Verification items for the finished model (mm, model axes). Coordinates: 2 decimals unless noted, no trailing zeros. Order: outer loops, then holes, each group sorted by start corner. A loop starts at its lowest first (then second) coordinate and runs counter-clockwise, first axis right, second up. Notation, with made-up numbers: M 53,28 L 73,28 A29 cw 73,54 Z; hole C 74.5,13.5 d2. An arc over 180 degrees is marked long. Return JSON: item names as keys, results as strings. Group by question number.
Q1. Thickness scan on probe 1 along Z at (x, y) = (-68, -8.25); probe 2 along X at (y, z) = (-7.25, 9); probe 3 along X at (y, z) = (-5.5, -53). Record the ranges inside material, lowest first.
Q2. Mould release check, pull along X, two halves, no side actions. Record for faces 1 (the face through (-106.14, -2.01, -52.54)), 2 (the face through (-97.832, -6.332, 43.282)), 3 (the face through (-66.504, -4.833, -28.468)): pulls with the +X half, pulls with the -X half, needs draft (parallel to the pull), parting line crosses it, or undercut.
Q3. Go/stop test with flat-tipped pins: pin 1 Ø1 at (x, y) = (-92.5, -5.5) entering from +Z; pin 2 Ø1.5 at (y, z) = (-1.5, -23) entering from +X. Record where each tip stops, or that it passes through.
Q4. Section check B-B, the plane y = -9.75. Enter the section's corners in (x, z).
Q5. Section check A-A, the plane y = -2.25. Enter the section's corners in (x, z), then the cut area to 3 significant figures.
from build123d import *

# Parameters (mm, degrees)
F0_R         = 57.9360533335
F2_DEPTH     = 12.7
F3_D         = 48.26
F5_D         = 33.02
F6_T2_ANGLE  = 283.4727948919
F6_T4_ANGLE  = 86.0712547595
F6_T6_ANGLE  = 107.4118170834
F6_T8_ANGLE  = 267.462303274
F6_T10_ANGLE = 277.2145700269
F6_T12_ANGLE = 103.4165555336
F6_T16_ANGLE = 107.4118170834
F6_T18_ANGLE = 283.4727948919
F6_T20_ANGLE = 277.2145700269
F6_T22_ANGLE = 86.0712547595
F6_T24_ANGLE = 103.4165555336
F6_T26_ANGLE = 267.462303274


# Not quite as in the source:
# - a fillet or chamfer that OpenCascade refuses, or shapes differently, is made with other operations: its cross-section is extruded or revolved along the edge and cut away or added


with BuildPart() as f2:
    # F0 (on Front) → F2 (new body)
    with BuildSketch(Plane.XZ):
        with Locations((-72.7998018265, -8.9674890041)):
            Circle(F0_R)
    extrude(amount=F2_DEPTH)

    # F3 (through all)
    with Locations(Plane(origin=(0, 0, 0), x_dir=(1, 0, 0), z_dir=(0, 1, 0))):
        with Locations((-45.7866154611, -28.1515028328), (-120.4445809126, 8.0565353855), (-60.4006908834, 52.0677864552)):
            Hole(F3_D / 2)

    # F5 (through all)
    with Locations(Plane(origin=(0, 0, 0), x_dir=(1, 0, 0), z_dir=(0, 1, 0))):
        with Locations((-74.9381706119, 4.8889117315)):
            Hole(F5_D / 2)

    # F6: chamfer of 5.08 on 14 edges, made by hand

    # F6_s1 → F6_t2 (revolve, cut)
    with BuildSketch(Plane(origin=(-33.5431340109, 0, 13.6983383479), x_dir=(0, 1, 0), z_dir=(0.9257774909, 0, -0.3780688263))):
        Polygon((-7.62, -95.1688030077), (-12.7, -100.2488030077), (-12.7, -95.1688030077), align=None)
    revolve(axis=Axis((-60.4006908834, -12.7, -52.0677864552), (0, 1, 0)), revolution_arc=F6_T2_ANGLE, mode=Mode.SUBTRACT)

    # F6_s3 → F6_t4 (revolve, cut)
    with BuildSketch(Plane(origin=(-0.6504253771, 0, 3.7035474889), x_dir=(0, 1, 0), z_dir=(-0.1729749681, 0, 0.9849262208))):
        Polygon((-12.7, 126.1096381457), (-7.62, 131.1896381457), (-12.7, 131.1896381457), align=None)
    revolve(axis=Axis((-72.7998018265, -12.7, -8.9674890041), (0, -1, 0)), revolution_arc=F6_T4_ANGLE, mode=Mode.SUBTRACT)

    # F6_s5 → F6_t6 (revolve, cut)
    with BuildSketch(Plane(origin=(-29.9879926822, 0, 31.6264228209), x_dir=(0, 1, 0), z_dir=(-0.6880604052, 0, 0.7256534151))):
        Polygon((-7.62, 1.0615455961), (-12.7, 6.1415455961), (-12.7, 1.0615455961), align=None)
    revolve(axis=Axis((-72.7998018265, -12.7, -8.9674890041), (0, 1, 0)), revolution_arc=F6_T6_ANGLE, mode=Mode.SUBTRACT)

    # F6_s7 → F6_t8 (revolve, cut)
    with BuildSketch(Plane(origin=(-69.201107614, 0, -63.7135426846), x_dir=(0, 1, 0), z_dir=(-0.7356739262, 0, -0.6773358652))):
        Polygon((-12.7, -104.8644514037), (-7.62, -99.7844514037), (-12.7, -99.7844514037), align=None)
    revolve(axis=Axis((-120.4445809126, -12.7, -8.0565353855), (0, 1, 0)), revolution_arc=F6_T8_ANGLE, mode=Mode.SUBTRACT)

    # F6_s9 → F6_t10 (revolve, cut)
    with BuildSketch(Plane(origin=(-8.1423267798, 0, 36.5399201696), x_dir=(0, 1, 0), z_dir=(-0.2174992035, 0, 0.9760604984))):
        Polygon((-12.7, 9.3575772605), (-7.62, 14.4375772605), (-12.7, 14.4375772605), align=None)
    revolve(axis=Axis((-45.7866154611, -12.7, 28.1515028328), (0, 1, 0)), revolution_arc=F6_T10_ANGLE, mode=Mode.SUBTRACT)

    # F6_s11 → F6_t12 (revolve, cut)
    with BuildSketch(Plane(origin=(-55.7502574842, 0, 26.6710376642), x_dir=(0, 1, 0), z_dir=(0.9020846433, 0, -0.4315591458))):
        Polygon((-12.7, 13.3491989235), (-7.62, 18.4291989235), (-12.7, 18.4291989235), align=None)
    revolve(axis=Axis((-72.7998018265, -12.7, -8.9674890041), (0, -1, 0)), revolution_arc=F6_T12_ANGLE, mode=Mode.SUBTRACT)

    # F6_s13 → F6_t14 (revolve, cut)
    with BuildSketch(Plane.XY.offset(-4.8889117315)):
        Polygon((-53.3481706119, -12.7), (-58.4281706119, -7.62), (-58.4281706119, -12.7), align=None)
    revolve(axis=Axis((-74.9381706119, -12.7, -4.8889117315), (0, 1, 0)), mode=Mode.SUBTRACT)

    # F6_s15 → F6_t16 (revolve, cut)
    with BuildSketch(Plane(origin=(-62.2843162467, 0, -30.4655418629), x_dir=(0, 1, 0), z_dir=(-0.8982965238, 0, -0.4393897533))):
        Polygon((-5.08, 34.004030567), (0, 28.924030567), (0, 34.004030567), align=None)
    revolve(axis=Axis((-72.7998018265, 0, -8.9674890041), (0, -1, 0)), revolution_arc=F6_T16_ANGLE, mode=Mode.SUBTRACT)

    # F6_s17 → F6_t18 (revolve, cut)
    with BuildSketch(Plane(origin=(-45.2248879791, 0, -62.9674495541), x_dir=(0, 1, 0), z_dir=(-0.5833556277, 0, -0.8122168501))):
        Polygon((0, 10.5255773581), (-5.08, 5.4455773581), (0, 5.4455773581), align=None)
    revolve(axis=Axis((-60.4006908834, 0, -52.0677864552), (0, -1, 0)), revolution_arc=F6_T18_ANGLE, mode=Mode.SUBTRACT)

    # F6_s19 → F6_t20 (revolve, cut)
    with BuildSketch(Plane(origin=(-8.1423267798, 0, 36.5399201696), x_dir=(0, 1, 0), z_dir=(-0.2174992035, 0, 0.9760604984))):
        Polygon((0, 9.3575772605), (-5.08, 14.4375772605), (0, 14.4375772605), align=None)
    revolve(axis=Axis((-45.7866154611, 0, 28.1515028328), (0, 1, 0)), revolution_arc=F6_T20_ANGLE, mode=Mode.SUBTRACT)

    # F6_s21 → F6_t22 (revolve, cut)
    with BuildSketch(Plane(origin=(-0.6504253771, 0, 3.7035474889), x_dir=(0, 1, 0), z_dir=(-0.1729749681, 0, 0.9849262208))):
        Polygon((0, 126.1096381457), (-5.08, 131.1896381457), (0, 131.1896381457), align=None)
    revolve(axis=Axis((-72.7998018265, 0, -8.9674890041), (0, -1, 0)), revolution_arc=F6_T22_ANGLE, mode=Mode.SUBTRACT)

    # F6_s23 → F6_t24 (revolve, cut)
    with BuildSketch(Plane(origin=(-55.7502574842, 0, 26.6710376642), x_dir=(0, 1, 0), z_dir=(0.9020846433, 0, -0.4315591458))):
        Polygon((0, 13.3491989235), (-5.08, 18.4291989235), (0, 18.4291989235), align=None)
    revolve(axis=Axis((-72.7998018265, 0, -8.9674890041), (0, -1, 0)), revolution_arc=F6_T24_ANGLE, mode=Mode.SUBTRACT)

    # F6_s25 → F6_t26 (revolve, cut)
    with BuildSketch(Plane(origin=(-56.5588266789, 0, 56.2173150628), x_dir=(0, 1, 0), z_dir=(-0.7092448082, 0, 0.7049622699))):
        Polygon((0, 119.832941055), (-5.08, 114.752941055), (0, 114.752941055), align=None)
    revolve(axis=Axis((-120.4445809126, 0, -8.0565353855), (0, -1, 0)), revolution_arc=F6_T26_ANGLE, mode=Mode.SUBTRACT)

    # F6_s27 → F6_t28 (revolve, cut)
    with BuildSketch(Plane.XY.offset(-4.8889117315)):
        Polygon((-53.3481706119, 0), (-58.4281706119, -5.08), (-58.4281706119, 0), align=None)
    revolve(axis=Axis((-74.9381706119, 0, -4.8889117315), (0, 1, 0)), mode=Mode.SUBTRACT)


solid = f2.part
Numbers:
{
 "1": {"probe 1": "z = -28.5 to -20.56, 10.78 to 17.21, 39.09 to 48.14", "probe 2": "x = -103.38 to -83.86, -66.01 to -60.47, -31.11 to -17.72", "probe 3": "x = -110.45 to -84.51, -36.29 to -35.15"},
 "2": {"face 1": "pulls with the -X half", "face 2": "parting line crosses it", "face 3": "undercut"},
 "3": {"pin 1": "stops at z = 45.69", "pin 2": "stops at x = -19.49"},
 "4": {"outline": "M -122.56,-34.23 A55.81 ccw -83.97,-63.64 A26.26 cw long -34.28,-49.35 A55.81 ccw -22.71,15.63 A26.26 cw -59.74,5.91 A18.64 cw long -66.12,11.53 A26.26 cw -64.8,46.26 A55.81 ccw -121.56,18.18 A26.26 cw long Z"},
 "5": {"outline": "M -121.37,-35 A55.11 ccw -85.19,-62.66 A26.96 cw long -33.77,-47.87 A55.11 ccw -22.76,14.12 A26.96 cw -57.76,4 A19.34 cw long -93.56,-10.1 A26.96 cw Z; M -120.34,18.9 A26.96 cw -94.1,-2.31 A19.34 cw -68.26,13.26 A26.96 cw -66.22,45.74 A55.11 ccw Z", "area": "3,880 mm2"}
}
